Autodesk Fusion 360 part; units mm, degrees
sketch "Bottom Access Panel" plane through (0, 0, 0) normal (0, 1, 0) x (1, 0, 0)
  line L0 (0, 0) -> (139, 0)
  line L1 (139, 0) -> (139, -139)
  line L2 (139, -139) -> (0, -139)
  line L3 (0, -139) -> (0, 0)
  dimension "d1" = 139
  dimension "d2" = 139
extrude "Extrude1" add sketch "Bottom Access Panel" along normal blind 6
fillet "Fillet1" radius 8 4 edges at (0, 3, 139) (139, 3, 139) (139, 3, 0) (0, 3, 0)
sketch "Magnet Holes" plane through (0, 0, 0) normal (0, 1, 0) x (1, 0, 0)
  arc A0 (8, 0) -> (0, -8) centre (8, -8) ccw
  line L0 (8, 0) -> (131, 0)
  arc A1 (139, -8) -> (131, 0) centre (131, -8) ccw
  line L1 (139, -8) -> (139, -131)
  arc A2 (131, -139) -> (139, -131) centre (131, -131) ccw
  line L2 (131, -139) -> (8, -139)
  arc A3 (0, -131) -> (8, -139) centre (8, -131) ccw
  line L3 (0, -131) -> (0, -8)
  circle A4 centre (9.5, -129.5) radius 2.75
  circle A5 centre (129.5, -129.5) radius 2.75
  circle A6 centre (9.5, -9.5) radius 2.75
  circle A7 centre (129.5, -9.5) radius 2.75
  dimension "d20" = 5.5
  dimension "d21" = 5.5
  dimension "d22" = 5.5
  dimension "d23" = 5.5
  dimension "d24" = 9.5
  dimension "d25" = 9.5
  dimension "d26" = 9.5
  dimension "d27" = 9.5
  dimension "d28" = 9.5
  dimension "d29" = 9.5
  dimension "d30" = 9.5
  dimension "d31" = 9.5
extrude "Extrude3" cut sketch "Magnet Holes" along normal blind 1.5 contours A4 | A5 | A6 | A7
equation "mdfThickness = 6 mm"
equation "d4 = mdfThickness"
equation "filletRadius = 8 mm"
equation "d15 = filletRadius"
Input: part model. Units: mm. Frame: model coordinates. A direction names the side the tool comes from. Give positions to 0.01 mm unless a question says otherwise; leave off trailing zeros.
Q1. Ray query, probe 1 along X at (y, z) = (0.95, 9.5); probe 2 along Z at (x, y) = (133, 5.6). Return the intervals inside material, ascending.
Checked values:
probe 1: x = 0 to 6.75, 12.25 to 126.75, 132.25 to 139
probe 2: z = 0.25 to 138.75
Q2. Contact query for flat-ended pins moving along their axis: pin 1 Ø6.5 at (x, z) = (9.5, 9.5) entering from -Y; pin 2 Ø5 at (x, z) = (9.5, 129.5) entering from -Y. Output: stop coordinate, or through.
Checked values:
pin 1: stops at y = 0
pin 2: stops at y = 1.5
Q3. Set-up query: faces 4 (the flat face through (69, 6, 69)), 5 (the cylindrical face through (130.77, 0.74, 127.06)). Return all of +Z, -Z, +X, -X, +Y, -Y with unobstructed straight access to the full face (end or side cutting, diameter ignored); none if empty.
Checked values:
face 4: +Z, -Z, +X, -X, +Y
face 5: -Y
Q4. Draft query along X for faces 1 (the flat face through (0, 3, 70)), 2 (the flat face through (69, 3, 0)), 3 (the cylindrical face through (9.142, 0.74, 12.227)). Return one class per face: +X half, -X half, draft (parallel to the pull), parting line (faces both ways), or undercut.
Checked values:
face 1: -X half
face 2: draft
face 3: undercut
